from build123d import *

# Parameters (mm, degrees)
EXTRUDE_1_DEPTH     = 15
SKETCH_2_W          = 18.78
SKETCH_2_H          = 26
EXTRUDE_2_DEPTH     = 20
SKETCH_3_W          = 8
SKETCH_3_H          = 54
EXTRUDE_3_DEPTH     = 5
SKETCH_4_W          = 8
SKETCH_4_H          = 20
EXTRUDE_4_DEPTH     = 30
CUT_EXTRUDE_2_DEPTH = 30
FILLET_1_R          = 6
FILLET_2_R          = 6
FILLET_3_R          = 7
FILLET_4_R          = 7
CHAMFER_1_SIZE      = 10
CHAMFER_2_SIZE      = 4
SKETCH_6_R          = 1.6
CUT_EXTRUDE_3_DEPTH = 179
SKETCH_9_W          = 20.537192292
SKETCH_9_H          = 20
CUT_EXTRUDE_4_DEPTH = 179
SKETCH_10_R         = 1.65
CUT_EXTRUDE_5_DEPTH = 179


with BuildPart() as part:
    # 草图1 → 凸台-拉伸1 (new body)
    with BuildSketch(Plane.XY):
        Polygon((0, 0), (8, 0), (8, 80), (30.14, 80), (30.14, 98), (-10.78, 98), (-10.78, 54), (0, 54), align=None)
    extrude(amount=EXTRUDE_1_DEPTH)

    # 草图2 → 凸台-拉伸2 (add)
    with BuildSketch(Plane.XY.offset(15)):
        with Locations((-1.39, 67)):
            Rectangle(SKETCH_2_W, SKETCH_2_H)
    extrude(amount=EXTRUDE_2_DEPTH)

    # 草图3 → 凸台-拉伸3 (add)
    with BuildSketch(Plane.XY.offset(15)):
        with Locations((4, 27)):
            Rectangle(SKETCH_3_W, SKETCH_3_H)
    extrude(amount=EXTRUDE_3_DEPTH)

    # 草图4 → 凸台-拉伸4 (add)
    with BuildSketch(Plane.XY.offset(20)):
        with Locations((4, 44)):
            Rectangle(SKETCH_4_W, SKETCH_4_H)
    extrude(amount=EXTRUDE_4_DEPTH)

    # 草图5 → 切除-拉伸2 (cut)
    with BuildSketch(Plane.XY.offset(15)):
        with BuildLine():
            Line((30.14, 90), (30.14, 91))
            Line((30.14, 91), (27.259215611, 91))
            ThreePointArc((27.259215611, 91), (18.98, 90), (27.259215611, 89))
            Line((27.259215611, 89), (30.14, 89))
            Line((30.14, 89), (30.14, 90))
        make_face()
    extrude(amount=-CUT_EXTRUDE_2_DEPTH, mode=Mode.SUBTRACT)

    # 圆角1
    fillet_1_edges = [part.edges().sort_by_distance(p)[0] for p in [
        (30.14, 98, 7.5),
    ]]
    fillet(fillet_1_edges, radius=FILLET_1_R)

    # 圆角2
    fillet_2_edges = [part.edges().sort_by_distance(p)[0] for p in [
        (30.14, 80, 7.5),
    ]]
    fillet(fillet_2_edges, radius=FILLET_2_R)

    # 圆角3
    fillet_3_edges = [part.edges().sort_by_distance(p)[0] for p in [
        (-10.78, 98, 7.5),
    ]]
    fillet(fillet_3_edges, radius=FILLET_3_R)

    # 圆角4
    fillet_4_edges = [part.edges().sort_by_distance(p)[0] for p in [
        (-10.78, 67, 35),
    ]]
    fillet(fillet_4_edges, radius=FILLET_4_R)

    # 倒角1
    chamfer_1_edges = [part.edges().sort_by_distance(p)[0] for p in [
        (4, 54, 35),
    ]]
    chamfer(chamfer_1_edges, length=CHAMFER_1_SIZE)

    # 倒角2
    chamfer_2_edges = [part.edges().sort_by_distance(p)[0] for p in [
        (0, 54, 17.5),
    ]]
    chamfer(chamfer_2_edges, length=CHAMFER_2_SIZE)

    # 草图6 → 切除-拉伸3 (cut)
    with BuildSketch(Plane(origin=(0, 80, 0), x_dir=(1, 0, 0), z_dir=(0, 1, 0))):
        with Locations((1.22, -25.05)):
            Circle(SKETCH_6_R)
    extrude(amount=-CUT_EXTRUDE_3_DEPTH, mode=Mode.SUBTRACT)

    # 草图9 → 切除-拉伸4 (cut)
    with BuildSketch(Plane.ZY):
        with Locations((30.268596146, 44)):
            Rectangle(SKETCH_9_W, SKETCH_9_H)
    extrude(amount=CUT_EXTRUDE_4_DEPTH, mode=Mode.SUBTRACT)

    # 草图10 → 切除-拉伸5 (cut)
    with BuildSketch(Plane.ZY):
        with Locations((40, 44)):
            Circle(SKETCH_10_R)
        with Locations((10, 10)):
            Circle(SKETCH_10_R)
        with Locations((10, 44)):
            Circle(SKETCH_10_R)
    extrude(amount=-CUT_EXTRUDE_5_DEPTH, mode=Mode.SUBTRACT)


solid = part.part
Here's how the part is built. I have some questions about the finished solid (model axes, mm). A direction names the side the tool comes from. Round coordinates to 2 decimals unless told otherwise and drop trailing zeros. Order: outer loops, then holes, each group sorted by start corner. A loop starts at its lowest first (then second) coordinate and runs counter-clockwise, first axis right, second up. Notation, with made-up numbers: M -30.75,-24 L 0.25,-24 A10 ccw 0.25,-15 Z; hole C 32,35.5 d8. An arc over 180 degrees is marked long. One line per question, with ' | ' between items.
1) I need wall thicknesses on line 1 (Y direction, x = 5, z = 10); line 2 (X direction, y = 54, z = 37.5); line 3 (Y direction, x = 23.18, z = 3.75). Which ranges of each line are inside material? Lowest first, please.
Checked values:
line 1: y = 0 to 8.35, 11.65 to 42.35, 45.65 to 98 | line 2: x = 0 to 8 | line 3: y = 80 to 85.8, 94.2 to 98
2) Imagine slicing it at D-D, the plane x = 23.18. Write out the boundary of the cut face in (y, z).
Checked values:
outline: M 80,0 L 85.8,0 L 85.8,15 L 80,15 Z; M 94.2,0 L 98,0 L 98,15 L 94.2,15 Z
3) I'm going to push flat-ended pins straight in: pin 1 Ø9 at (x, y) = (3.5, 12) entering from +Z; pin 2 Ø0.9 at (x, z) = (28.5, 6.5) entering from +Y; pin 3 Ø5.5 at (y, z) = (10, 10) entering from +X; pin 4 Ø2.5 at (x, z) = (1.22, 25.05) entering from +Y. Where does each tip first touch, or does it pass through?
Checked values:
pin 1: stops at z = 20 | pin 2: stops at y = 96.55 | pin 3: stops at x = 8 | pin 4: passes through
4) We'd pull the mould along Z, two halves only. Please class faces 1 (the cylindrical face through (3.944, 45.115, 38.784)), 2 (the flat face through (8, 48, 19)), 3 (the cylindrical face through (2.746, 57.322, 24.569)), 4 (the flat face through (4, 59, 40)): released by +Z, released by -Z, zero draft, split by the parting line, or undercut.
Checked values:
face 1: undercut | face 2: zero draft | face 3: undercut | face 4: released by +Z
5) On a 3-axis mill with a long thin cutter (end or side, diameter ignored), from which of +Z, -Z, +X, -X, +Y, -Y can I reach the whole of each face in a straight line? I mean faces 5 (the flat face through (4, 54, 47)), 6 (the flat face through (4, 44, 50)), 7 (the flat face through (4, 17, 20)), 8 (the flat face through (29, 89, 8)), 9 (the flat face through (16, 80, 7)). Say none if no direction works.
Checked values:
face 5: +Z, +X, -X, +Y | face 6: +Z, +X, -X, +Y, -Y | face 7: +Z, +X, -X, -Y | face 8: +Z, -Z, +X | face 9: +Z, -Z, +X, -Y
6) Imagine slicing it at B-B, the plane x = 1.22. Write out the boundary of the cut face in (y, z), plus the area to 3 significant figures.
Checked values:
outline: M 0,0 L 98,0 L 98,15 L 80,15 L 80,23.45 L 34,23.45 L 34,20 L 0,20 Z; M 34,26.65 L 80,26.65 L 80,35 L 64,35 L 54,45 L 54,50 L 34,50 Z; hole C 10,10 d3.3; hole C 44,10 d3.3; hole C 44,40 d3.3 | area: 2,740 mm²
7) Imagine slicing it at C-C, the plane y = 44. Write out the boundary of the cut face in (x, z), plus the area to 3 significant figures.
Checked values:
outline: M 0,0 L 8,0 L 8,8.35 L 0,8.35 Z; M 0,11.65 L 8,11.65 L 8,38.35 L 0,38.35 L 0,26.09 A1.6 cw long 0,24.01 Z; M 0,41.65 L 8,41.65 L 8,50 L 0,50 Z | area: 340 mm²
8) Imagine slicing it at A-A, the plane z = 25.05. Write out the boundary of the cut face in (x, y), plus the area to 3 significant figures.
Checked values:
outline: M -10.78,54 L -0.38,54 L -0.38,80 L -10.78,80 Z; M 2.82,34 L 8,34 L 8,80 L 2.82,80 Z | area: 509 mm²
